from build123d import *

# Parameters (mm, degrees)
BOSS_EXTRUDE1_DEPTH = 500


with BuildPart() as part:
    # Sketch1 → Boss-Extrude1 (new body)
    with BuildSketch(Plane.XY):
        with BuildLine():
            Line((1.5, -18.3), (15, -18.3))
            Line((15, -18.3), (15, -22.3))
            Line((15, -22.3), (-15, -22.3))
            Line((-15, -22.3), (-15, -18.3))
            Line((-15, -18.3), (-1.5, -18.3))
            Line((-1.5, -18.3), (-1.5, -5.809475019))
            ThreePointArc((-1.5, -5.809475019), (0, 6), (1.5, -5.809475019))
            Line((1.5, -5.809475019), (1.5, -18.3))
        make_face()
    extrude(amount=BOSS_EXTRUDE1_DEPTH)


solid = part.part
Source: CAD feature listing. Evaluate the final solid. Frame: model axes, mm. A direction names the side the tool comes from. Coordinates: 2 decimals unless noted, no trailing zeros. Loops run counter-clockwise (first coordinate to the right, second up) from the corner with the lowest first, then second, coordinate; pieces in that order, holes last. Notation, with made-up numbers: (29, 52.5) - (50, 52.5) arc R10 cw to (50, 67.5) - close; hole circle Ø1 at (-6.5, -31.5). An arc over 180 degrees is marked (long way). One line per question, with ' | ' between items.
1) Section A-A, the plane z = 467.5. Return loops of the section in (x, y), then the cut area to 3 significant figures.
Report:
outline: (-15, -22.3) - (15, -22.3) - (15, -18.3) - (1.5, -18.3) - (1.5, -5.81) arc R6 ccw (long way) to (-1.5, -5.81) - (-1.5, -18.3) - (-15, -18.3) - close | area: 270 mm²
2) Section B-B, the plane y = -11.25. Return loops of the section in (x, z), then the cut area to 3 significant figures.
Report:
outline: (-1.5, 0) - (1.5, 0) - (1.5, 500) - (-1.5, 500) - close | area: 1,500 mm²
3) Pull-direction query (Y, two-part tool) for faces 4 (the face through (0, -22.3, 246)), 5 (the face through (1, -10, 0)), 6 (the face through (-1.5, -12, 246)); classes: released by +Y, released by -Y, zero draft, split by the parting line, or undercut.
Report:
face 4: released by -Y | face 5: zero draft | face 6: undercut
4) Line query: line 1 along X through (y, z) = (-16.25, 395.5); line 2 along Y through (x, z) = (-0.25, 358); line 3 along Y through (x, z) = (-7, 243). Output: solid intervals per line, ascending.
Report:
line 1: x = -1.5 to 1.5 | line 2: y = -22.3 to 5.99 | line 3: y = -22.3 to -18.3
5) First-contact query: P1, Ø11, axis at x = -7.5, z = 320, coming from the +Y side; P2, Ø2, axis at x = 2.5, z = 268.5, coming from the +Y side; P3, Ø6, axis at y = -14, z = 376, coming from the +X side. Flat tips, straight axial feed; report the tip coordinate or a pass-through.
Report:
P1: stops at y = 5.66 | P2: stops at y = 5.81 | P3: stops at x = 1.5
6) Set-up query: faces 1 (the face through (-8, -18.3, 246)), 2 (the face through (0, 6, 246)), 3 (the face through (1.5, -12, 246)). Return all of +Z, -Z, +X, -X, +Y, -Y with unobstructed straight access to the full face (end or side cutting, diameter ignored); none if empty.
Report:
face 1: +Z, -Z, -X | face 2: +Z, -Z | face 3: +Z, -Z, +X
